from build123d import *

# Parameters (mm, degrees)
SALIENTE_EXTRUIR1_DEPTH = 60
CROQUIS2_W              = 5
CROQUIS2_H              = 41
CORTAR_EXTRUIR1_DEPTH   = 20
CROQUIS7_R              = 2.2
CROQUIS7_R_2            = 2.253524607
CORTAR_EXTRUIR5_DEPTH   = 10
CROQUIS8_R              = 1.5
CORTAR_EXTRUIR6_DEPTH   = 10
CROQUIS9_R              = 4
CROQUIS9_R_2            = 1.621314805
CORTAR_EXTRUIR7_DEPTH   = 3
CROQUIS10_R             = 1.621314805
CORTAR_EXTRUIR8_DEPTH   = 10


with BuildPart() as part:
    # Croquis1 → Saliente-Extruir1 (new body)
    with BuildSketch(Plane.XY):
        Polygon((0, 0), (40, 0), (40, 5), (31, 5), (31, 25), (26, 25), (26, 5), (5, 5), (5, 30), (0, 30), align=None)
    extrude(amount=SALIENTE_EXTRUIR1_DEPTH)

    # Croquis2 → Cortar-Extruir1 (cut)
    with BuildSketch(Plane(origin=(0, 25, 0), x_dir=(1, 0, 0), z_dir=(0, 1, 0))):
        with Locations((28.5, -30)):
            Rectangle(CROQUIS2_W, CROQUIS2_H)
    extrude(amount=-CORTAR_EXTRUIR1_DEPTH, mode=Mode.SUBTRACT)

    # Croquis7 → Cortar-Extruir5 (cut)
    with BuildSketch(Plane(origin=(31, 0, 0), x_dir=(0, 0, -1), z_dir=(1, 0, 0))):
        with Locations(Location((-53.9, 20.1, 0), (0, 0, 90))):
            Circle(CROQUIS7_R)
        with Locations(Location((-53.9, 9.9, 0), (0, 0, 90))):
            Circle(CROQUIS7_R)
        with Locations(Location((-6.1, 9.9, 0), (0, 0, 90))):
            Circle(CROQUIS7_R)
        with Locations(Location((-6.1, 20.1, 0), (0, 0, 90))):
            Circle(CROQUIS7_R_2)
    extrude(amount=-CORTAR_EXTRUIR5_DEPTH, mode=Mode.SUBTRACT)

    # Croquis8 → Cortar-Extruir6 (cut)
    with BuildSketch(Plane.ZY):
        with Locations(Location((20, 15, 0), (0, 0, 270))):
            Circle(CROQUIS8_R)
        with Locations(Location((38.208996139, 15, 0), (0, 0, 270))):
            Circle(CROQUIS8_R)
    extrude(amount=-CORTAR_EXTRUIR6_DEPTH, mode=Mode.SUBTRACT)

    # Croquis9 → Cortar-Extruir7 (cut)
    with BuildSketch(Plane(origin=(5, 0, 0), x_dir=(0, 0, -1), z_dir=(1, 0, 0))):
        with Locations(Location((-20, 15, 0), (0, 0, 90))):
            Circle(CROQUIS9_R)
        with Locations(Location((-29.104498069, 15, 0), (0, 0, 90))):
            Circle(CROQUIS9_R_2)
        with Locations(Location((-38.208996139, 15, 0), (0, 0, 90))):
            Circle(CROQUIS9_R)
    extrude(amount=-CORTAR_EXTRUIR7_DEPTH, mode=Mode.SUBTRACT)

    # Croquis10 → Cortar-Extruir8 (cut)
    with BuildSketch(Plane(origin=(2, 0, 0), x_dir=(0, 0, -1), z_dir=(1, 0, 0))):
        with Locations(Location((-29.104498069, 15, 0), (0, 0, 90))):
            Circle(CROQUIS10_R)
    extrude(amount=-CORTAR_EXTRUIR8_DEPTH, mode=Mode.SUBTRACT)


solid = part.part
CAD build for the part. Positions are in the model's coordinates, mm. A direction names the side the tool comes from. Give positions to 0.01 mm unless a question says otherwise; leave off trailing zeros. Loops run counter-clockwise (first coordinate to the right, second up) from the corner with the lowest first, then second, coordinate; pieces in that order, holes last. Notation, with made-up numbers: M 69,-28 L 118,-28 A35 cw 118,4 Z; hole C 56,72.5 d6. An arc over 180 degrees is marked long. Answer in a Markdown table with one row per item. Add a question column.
Item 1: Probe probe 1 along Z at (x, y) = (27.55, 20.1); probe 2 along Z at (x, y) = (1.5, 15); probe 3 along X at (y, z) = (6.75, 7.5). List the from-to ranges inside material, lowest first.
Item 2: Band-saw the part on C-C on y = 15. Give the number of separate pieces and of enclosed holes in the cut face, then the cut area to 3 significant figures.
Item 3: Drop flat-ended pins along their axis: P1, Ø4, axis at y = 14.5, z = 20, coming from the +X side; P2, Ø5, axis at y = 16, z = 3.5, coming from the +X side; P3, Ø1.5, axis at x = 28.5, z = 56.5, coming from the +Y side. Give the stop position or say it passes through.
Item 4: Tool access for faces 4 (the face through (26, 15, 5)), 5 (the face through (29, 25, 55)), 6 (the face through (28, 15, 9.5)), 7 (the face through (0, 19, 30)), 8 (the face through (2, 17, 38)): list every direction of +Z, -Z, +X, -X, +Y, -Y with a clear straight run to the whole face (end or side of a thin tool).
Item 5: Band-saw the part on B-B on z = 6.1. Give the cut face in (x, y).
Item 6: Mould opens along Z. For faces 1 (the face through (31, 15, 55)), 2 (the face through (28.54, 22.25, 6.78)), 3 (the face through (17, 4, 0)) say: +Z half, -Z half, draft (parallel to the pull), parting line (faces both ways), or undercut.
Item 7: Band-saw the part on A-A on y = 9.9. Give the cut face in (x, z).
Item 8: Band-saw the part on D-D on y = 6.5. Give the cut face in (x, z).
Reply:
| question | item | result |
|---|---|---|
| 1 | probe 1 | z = 0 to 3.85, 8.35 to 9.5, 50.5 to 51.7, 56.1 to 60 |
| 1 | probe 2 | z = 0 to 18.5, 21.5 to 27.48, 30.73 to 36.71, 39.71 to 60 |
| 1 | probe 3 | x = 0 to 5, 26 to 31 |
| 2 | separate pieces | 6 |
| 2 | enclosed holes | 0 |
| 2 | area | 319 mm^2 |
| 3 | P1 | stops at x = 2 |
| 3 | P2 | stops at x = 31 |
| 3 | P3 | stops at y = 25 |
| 4 | face 4 | +Z, -Z, +Y |
| 4 | face 5 | +Z, -Z, +X, +Y |
| 4 | face 6 | +X, +Y |
| 4 | face 7 | +Z, -Z, -X, +Y, -Y |
| 4 | face 8 | +X |
| 5 | outline | M 0,0 L 40,0 L 40,5 L 31,5 L 31,7.7 L 26,7.7 L 26,5 L 5,5 L 5,30 L 0,30 Z; M 26,12.1 L 31,12.1 L 31,17.85 L 26,17.85 Z; M 26,22.35 L 31,22.35 L 31,25 L 26,25 Z |
| 6 | face 1 | draft |
| 6 | face 2 | undercut |
| 6 | face 3 | -Z half |
| 7 | outline | M 0,0 L 5,0 L 5,60 L 0,60 Z; M 26,0 L 31,0 L 31,3.9 L 26,3.9 Z; M 26,8.3 L 31,8.3 L 31,9.5 L 26,9.5 Z; M 26,50.5 L 31,50.5 L 31,51.7 L 26,51.7 Z; M 26,56.1 L 31,56.1 L 31,60 L 26,60 Z |
| 8 | outline | M 0,0 L 5,0 L 5,60 L 0,60 Z; M 26,0 L 31,0 L 31,9.5 L 26,9.5 Z; M 26,50.5 L 31,50.5 L 31,60 L 26,60 Z |
